Build history of the part. All positions in model axes, mm. A direction names the side the tool comes from. Round coordinates to 2 decimals unless told otherwise and drop trailing zeros. Order: outer loops, then holes, each group sorted by start corner. A loop starts at its lowest first (then second) coordinate and runs counter-clockwise, first axis right, second up. Notation, with made-up numbers: (52.5, -24) -> (81.5, -24) arc R33 cw to (81.5, 10) -> close; hole circle Ø4 at (70.25, -30.75). An arc over 180 degrees is marked (long way). Answer as a JSON object with one key per item and string values.
Autodesk Inventor part; units mm, degrees
ref_plane "YZ Plane" through (0, 0, 0) normal (1, 0, 0) x (0, 1, 0)
ref_plane "XZ Plane" through (0, 0, 0) normal (0, 1, 0) x (-1, 0, 0)
ref_plane "XY Plane" through (0, 0, 0) normal (0, 0, 1) x (1, 0, 0)
sketch "Sketch1" plane through (0, 0, 0) normal (1, 0, 0) x (0, 1, 0)
  line L0 (104, 124.9907) -> (104, 66.293)
  line L1 (239.8243, 220.0959) -> (104, 124.9907)
  line L2 (227.1683, 205.1302) -> (109, 122.3878)
  line L3 (109, 122.3878) -> (109, 66.293)
  line L4 (144.9576, 153.6695) -> (147.8255, 149.5737)
  line L5 (109, 66.293) -> (104, 66.293)
  point P0 (0, 0)
  dimension "d2" = 58.6977
  dimension "d3" = 50
extrude "Extrusion1" add sketch "Sketch1" along normal blind 43
properties part number "shooter bracket without motor"
1) Cut at A-A, the plane x = 20. Give the cut face in (y, z).
Checked values:
{"outline": "(104, 66.29) -> (109, 66.29) -> (109, 122.39) -> (147.83, 149.57) -> (144.96, 153.67) -> (104, 124.99) -> close"}
2) Probe L1, parallel to Y at x = 30, z = 99; L2, parallel to Z at x = 38, y = 118.5; L3, parallel to Z at x = 37, y = 112. List the from-to ranges inside material, lowest first. Write a range as from..to.
Checked values:
{"L1": "y = 104..109", "L2": "z = 129.04..135.14", "L3": "z = 124.49..130.59"}
3) Which spindle directions (+Z, -Z, +X, -X, +Y, -Y) get a long thin tool onto all of the face, cutting with end or side? Do faces 1 (the face through (21, 104, 96)), 2 (the face through (21, 109, 95)). Say none if no direction does.
Checked values:
{"face 1": "+Z, -Z, +X, -X, -Y", "face 2": "-Z, +X, -X, +Y"}
4) Flat gauge pins, fed straight in: pin 1 Ø13 at (x, z) = (11.5, 99.5) entering from +Y; pin 2 Ø1 at (x, y) = (12, 122) entering from -Z; pin 3 Ø1 at (x, z) = (9, 129) entering from +Y. Where does each tip first touch, or does it go through?
Checked values:
{"pin 1": "stops at y = 109", "pin 2": "stops at z = 131.14", "pin 3": "stops at y = 119.16"}
5) Cut at C-C, the plane y = 116. Give the cut face in (x, z), plus the area to 3 significant figures.
Checked values:
{"outline": "(0, 127.29) -> (43, 127.29) -> (43, 133.39) -> (0, 133.39) -> close", "area": "262 mm²"}
6) Cut at B-B, the plane z = 101. Give the cut face in (x, y), plus the area to 3 significant figures.
Checked values:
{"outline": "(0, 104) -> (43, 104) -> (43, 109) -> (0, 109) -> close", "area": "215 mm²"}
